Geometry check sheet. Reference: drawing and pictorial views, mm from the part's lowest x, y, z. Round coordinates to 2 decimals unless told otherwise and drop trailing zeros. Order: outer loops, then holes, each group sorted by start corner. A loop starts at its lowest first (then second) coordinate and runs counter-clockwise, first axis right, second up. Notation, with made-up numbers: (27.25, 46.25) -> (35.25, 46.25) arc R29 cw to (35.25, 66.25) -> close; hole circle Ø1 at (73.25, 67.5). An arc over 180 degrees is marked (long way). Put each result on its own line as item: value.
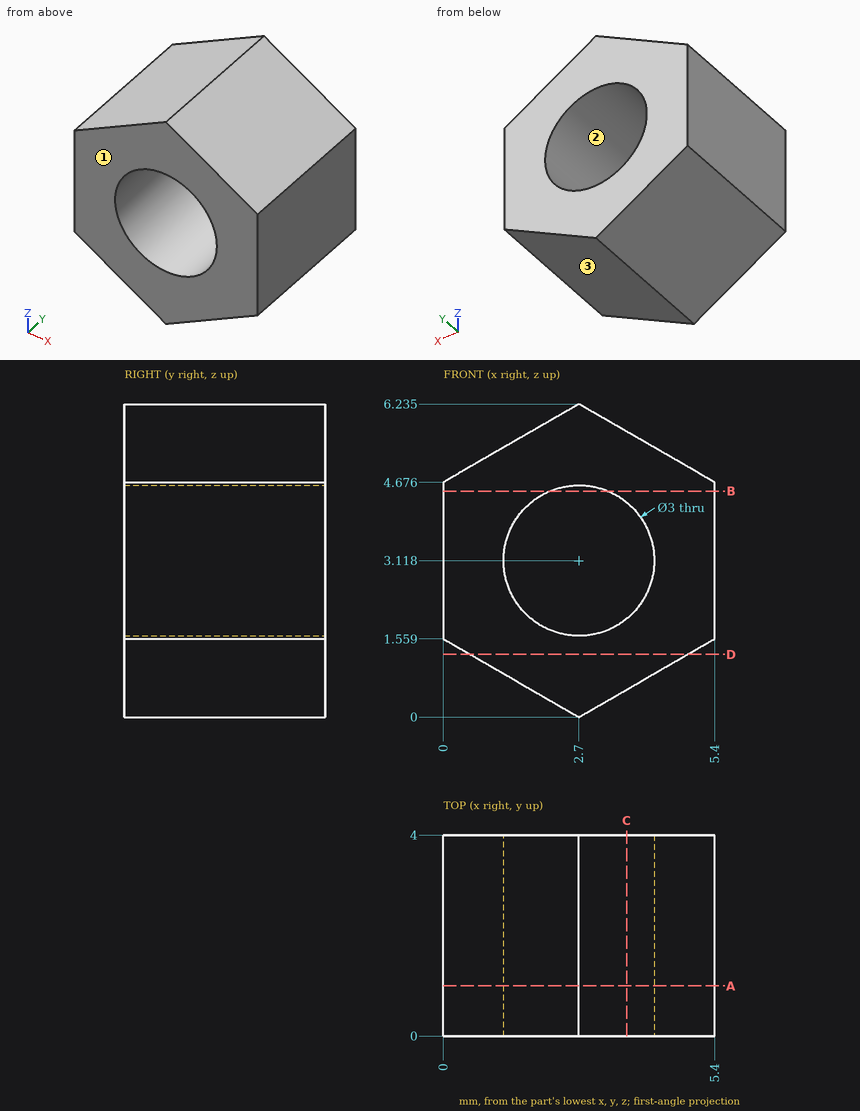
Item 1: Depth check by flat-ended pin: pin 1 Ø1 at (y, z) = (1.5, 1) entering from -X (1 decimal); pin 2 Ø1.5 at (x, y) = (4, 2) entering from -Z. Enter the tip coordinate at first touch or a pass-through.
Geometry check:
pin 1: x = 0.1
pin 2: z = 0.32
Item 2: Sectioned sample at A-A, the plane y = 1. Record the boundary of the cut face in (x, z) (1 decimal), then the cut area to 3 significant figures.
Geometry check:
outline: (0, 1.6) -> (2.7, 0) -> (5.4, 1.6) -> (5.4, 4.7) -> (2.7, 6.2) -> (0, 4.7) -> close; hole circle Ø3 at (2.7, 3.1)
area: 18.2 mm2
Item 3: Release check for a two-part mould opening along X. For the marked faces 1, 2 and 3 record: pulls with the +X half, pulls with the -X half, needs draft (parallel to the pull), parting line crosses it, or undercut.
Geometry check:
face 1: needs draft
face 2: undercut
face 3: pulls with the +X half
Item 4: Material ranges on line 1 along X through (y, z) = (3.05, 3.25) (1 decimal); line 2 along Z through (x, y) = (3.3, 0.7) (1 decimal); line 3 along X through (y, z) = (0.7, 2.5) (1 decimal), recorded low to high.
Geometry check:
line 1: 0 to 1.2, 4.2 to 5.4
line 2: 0.3 to 1.7, 4.5 to 5.9
line 3: 0 to 1.3, 4.1 to 5.4
Item 5: Sectioned sample at D-D, the plane z = 1.25. Record the boundary of the cut face in (x, y) (1 decimal).
Geometry check:
outline: (0.5, 0) -> (4.9, 0) -> (4.9, 4) -> (0.5, 4) -> close
Item 6: Sectioned sample at B-B, the plane z = 4.5. Record the boundary of the cut face in (x, y).
Geometry check:
outline: (0, 0) -> (2.12, 0) -> (2.12, 4) -> (0, 4) -> close; (3.28, 0) -> (5.4, 0) -> (5.4, 4) -> (3.28, 4) -> close
Item 7: Sectioned sample at C-C, the plane x = 3.65. Record the boundary of the cut face in (y, z).
Geometry check:
outline: (0, 0.55) -> (4, 0.55) -> (4, 1.96) -> (0, 1.96) -> close; (0, 4.28) -> (4, 4.28) -> (4, 5.69) -> (0, 5.69) -> close
